Input: part model. Units: mm. Frame: model coordinates. Face numbers are marked on the shaded views. A direction names the side the tool comes from. Give positions to 0.01 mm unless a question says otherwise; leave off trailing zeros. Loops run counter-clockwise (first coordinate to the right, second up) from the corner with the lowest first, then second, coordinate; pieces in that order, holes last. Notation, with made-up numbers: (82, 35) -> (93, 35) arc R16 cw to (93, 47) -> close; hole circle Ø2 at (-28, 25). An arc over 180 degrees is marked (long way). Answer as a JSON object with one key per item and string values.
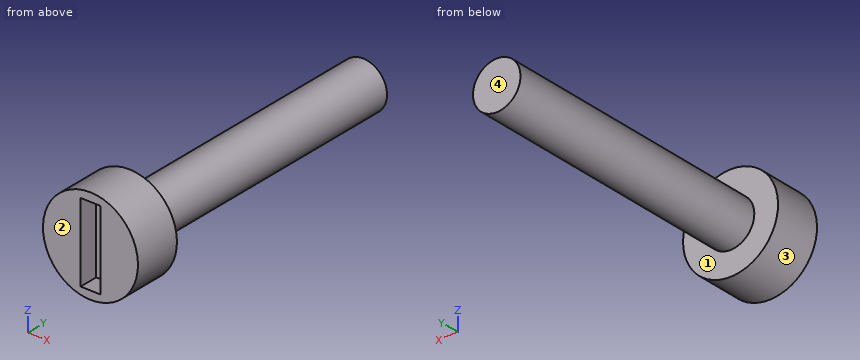
```python
from build123d import *

# Parameters (mm, degrees)
SKETCH_1_R          = 5
EXTRUDE_1_DEPTH     = 5
SKETCH_2_R          = 2.5
EXTRUDE_2_DEPTH     = 30
SKETCH_3_W          = 2.0741403
SKETCH_3_H          = 8.233435191
CUT_EXTRUDE_1_DEPTH = 2


with BuildPart() as part:
    # 草图1 → 凸台-拉伸1 (new body)
    with BuildSketch(Plane(origin=(0, 0, 0), x_dir=(1, 0, 0), z_dir=(0, 1, 0))):
        with Locations(Location((0, 0, 0), (0, 0, 270))):
            Circle(SKETCH_1_R)
    extrude(amount=EXTRUDE_1_DEPTH)

    # 草图2 → 凸台-拉伸2 (add)
    with BuildSketch(Plane(origin=(0, 5, 0), x_dir=(1, 0, 0), z_dir=(0, 1, 0))):
        with Locations(Location((0, 0, 0), (0, 0, 270))):
            Circle(SKETCH_2_R)
    extrude(amount=EXTRUDE_2_DEPTH)

    # 草图3 → 切除-拉伸1 (cut)
    with BuildSketch(Plane.XZ):
        with Locations((0, -0.009018001)):
            Rectangle(SKETCH_3_W, SKETCH_3_H)
    extrude(amount=-CUT_EXTRUDE_1_DEPTH, mode=Mode.SUBTRACT)


solid = part.part
```
Q1. Section A-A, the plane x = 0. Return the cut outline in (y, z).
Evaluation:
{"outline": "(0, -5) -> (5, -5) -> (5, -2.5) -> (35, -2.5) -> (35, 2.5) -> (5, 2.5) -> (5, 5) -> (0, 5) -> (0, 4.11) -> (2, 4.11) -> (2, -4.13) -> (0, -4.13) -> close"}
Q2. Section C-C, the plane y = 21. Return the cut outline in (x, z).
Evaluation:
{"outline": "circle Ø5 at (0, 0)"}
Q3. Section D-D, the plane x = 2. Return the cut outline in (y, z).
Evaluation:
{"outline": "(0, -4.58) -> (5, -4.58) -> (5, -1.5) -> (35, -1.5) -> (35, 1.5) -> (5, 1.5) -> (5, 4.58) -> (0, 4.58) -> close"}
Q4. Access query for the marked faces 1 and 2. Directions: +Z, -Z, +X, -X, +Y, -Y. A direction counts if a zero-diameter tool reaches every point of the face in a straight line with its end or side. Return the directions, or none.
Evaluation:
{"face 1": "+Y", "face 2": "+Z, -Z, +X, -X, -Y"}
Q5. Pin query (flat end, axial travel): pin 1 (1 mm diameter, centred on x = -1.5, y = 7.5, fed in from +Z); pin 2 (1 mm diameter, centred on y = 30, z = 1.5, fed in from -X); pin 3 (1.6 mm diameter, centred on y = 0.5, z = -2, fed in from +X). Return the tip coordinate at first contact, or that it passes through.
Evaluation:
{"pin 1": "stops at z = 2.29", "pin 2": "stops at x = -2.29", "pin 3": "stops at x = 4.85"}
Q6. Draft query along X for the marked faces 3 and 4. Return one class per face: +X half, -X half, draft (parallel to the pull), parting line (faces both ways), or undercut.
Evaluation:
{"face 3": "parting line", "face 4": "draft"}
Q7. Section B-B, the plane z = 0. Return the cut outline in (x, y).
Evaluation:
{"outline": "(-5, 0) -> (-1.04, 0) -> (-1.04, 2) -> (1.04, 2) -> (1.04, 0) -> (5, 0) -> (5, 5) -> (2.5, 5) -> (2.5, 35) -> (-2.5, 35) -> (-2.5, 5) -> (-5, 5) -> close"}
Q8. Ray query, line 1 along Y through (x, z) = (-3.5, -3.5); line 2 along Y through (x, z) = (0.5, 3.75); line 3 along X through (y, z) = (15, 0). Return the intervals inside material, ascending.
Evaluation:
{"line 1": "y = 0 to 5", "line 2": "y = 2 to 5", "line 3": "x = -2.5 to 2.5"}
